Read the model definition and answer for the solid it produces. Units are mm, in the model's axes. A direction names the side the tool comes from. Coordinates: 2 decimals unless noted, no trailing zeros. Order: outer loops, then holes, each group sorted by start corner. A loop starts at its lowest first (then second) coordinate and runs counter-clockwise, first axis right, second up. Notation, with made-up numbers: M 3.25,-23 L 55.25,-23 A20 cw 55.25,-12 Z; hole C 31,-37 d1. An arc over 180 degrees is marked long. Write each question's results on one line, items separated by ' | '.
```python
from build123d import *

# Parameters (mm, degrees)
F0_W           = 29
F0_H           = 35
F0_R           = 1.15
F0_W_2         = 19
F0_H_2         = 25
F1_DEPTH       = 6.5
F2_W           = 29
F2_H           = 35
F2_R           = 1.15
F2_W_2         = 19
F2_H_2         = 25
F3_DEPTH       = 4
F4_W           = 11
F4_H           = 5
F4_W_2         = 5
F5_DEPTH       = 6
F6_R           = 2
F8_D           = 2.9
F8_CBORE_D     = 5.5
F8_CBORE_DEPTH = 2.5


with BuildPart() as f1:
    # F0 (on Top) → F1 (new body)
    with BuildSketch(Plane.XY):
        Rectangle(F0_W, F0_H)
        with Locations((-12, -15)):
            Circle(F0_R, mode=Mode.SUBTRACT)
        with Locations((12, -15)):
            Circle(F0_R, mode=Mode.SUBTRACT)
        with Locations((-12, 15)):
            Circle(F0_R, mode=Mode.SUBTRACT)
        Rectangle(F0_W_2, F0_H_2, mode=Mode.SUBTRACT)
        with Locations((12, 15)):
            Circle(F0_R, mode=Mode.SUBTRACT)
    extrude(amount=F1_DEPTH)

    # F2 (on face) → F3 (join)
    with BuildSketch(Plane(origin=(0, 0, 0), x_dir=(1, 0, 0), z_dir=(0, 0, -1))):
        Rectangle(F2_W, F2_H)
        with Locations((-12, -15)):
            Circle(F2_R, mode=Mode.SUBTRACT)
        with Locations((12, -15)):
            Circle(F2_R, mode=Mode.SUBTRACT)
        with Locations((-12, 15)):
            Circle(F2_R, mode=Mode.SUBTRACT)
        Rectangle(F2_W_2, F2_H_2, mode=Mode.SUBTRACT)
        with Locations((12, 15)):
            Circle(F2_R, mode=Mode.SUBTRACT)
        with Locations((-12, 15)):
            Circle(F2_R)
        with Locations((12, 15)):
            Circle(F2_R)
        with Locations((-12, -15)):
            Circle(F2_R)
        Rectangle(F2_W_2, F2_H_2)
        with Locations((12, -15)):
            Circle(F2_R)
    extrude(amount=F3_DEPTH)

    # F4 (on face) → F5 (cut)
    with BuildSketch(Plane.XY.offset(6.5)):
        with Locations((0, -15)):
            Rectangle(F4_W, F4_H)
        with Locations((0, 15)):
            Rectangle(F4_W_2, F4_H)
    extrude(amount=-F5_DEPTH, mode=Mode.SUBTRACT)

    # F6
    f6_edges = [f1.edges().sort_by_distance(p)[0] for p in [
        (-14.5, 17.5, 1.25),
        (14.5, 17.5, 1.25),
        (14.5, -17.5, 1.25),
        (-14.5, -17.5, 1.25),
    ]]
    fillet(f6_edges, radius=F6_R)

    # F8 (through all)
    with Locations(Plane.XY):
        with Locations((0, 7), (0, -7)):
            CounterBoreHole(F8_D / 2, F8_CBORE_D / 2, F8_CBORE_DEPTH)


solid = f1.part
```
(1) The part is cut by section A-A, the plane z = 2.75. Write down the section's boundary in (x, y), then the cut area to 3 significant figures.
Conclusion:
outline: M -14.5,-15.5 A2 ccw -12.5,-17.5 L -5.5,-17.5 L -5.5,-12.5 L -9.5,-12.5 L -9.5,12.5 L -2.5,12.5 L -2.5,17.5 L -12.5,17.5 A2 ccw -14.5,15.5 Z; M 2.5,12.5 L 9.5,12.5 L 9.5,-12.5 L 5.5,-12.5 L 5.5,-17.5 L 12.5,-17.5 A2 ccw 14.5,-15.5 L 14.5,15.5 A2 ccw 12.5,17.5 L 2.5,17.5 Z; hole C -12,-15 d2.3; hole C -12,15 d2.3; hole C 12,-15 d2.3; hole C 12,15 d2.3 | area: 440 mm²
(2) The part is cut by section B-B, the plane y = -7. Write down the section's boundary in (x, z), then the cut area to 3 significant figures.
Conclusion:
outline: M -14.5,-4 L -1.45,-4 L -1.45,-2.5 L -2.75,-2.5 L -2.75,0 L -9.5,0 L -9.5,6.5 L -14.5,6.5 Z; M 1.45,-4 L 14.5,-4 L 14.5,6.5 L 9.5,6.5 L 9.5,0 L 2.75,0 L 2.75,-2.5 L 1.45,-2.5 Z | area: 163 mm²
(3) Straight lines are drawn through the part: line 1 (Y direction, x = 0, z = -3.4); line 2 (Y direction, x = 0, z = -1.15); line 3 (Y direction, x = 6.75, z = 2.25). For each, find the intervals that lie inside material, in ascending order.
Conclusion:
line 1: -17.5 to -8.45, -5.55 to 5.55, 8.45 to 17.5 | line 2: -17.5 to -9.75, -4.25 to 4.25, 9.75 to 17.5 | line 3: -17.5 to -12.5, 12.5 to 17.5
(4) For faces 1 (the flat face through (0, 15, 0.5)), 2 (the flat face through (1.2, -8.2, -2.5)), 3 (the flat face through (-5.5, -15, 4)), determine the directions among +Z, -Z, +X, -X, +Y, -Y from which every point of the face is accessible in a straight line to the end or side of a thin tool.
Conclusion:
face 1: +Z, +Y, -Y | face 2: +Z | face 3: +Z, -Y
(5) Given pin 1 (4.5 mm diameter, centred on x = 0, y = 7, fed in from +Z); pin 2 (1.1 mm diameter, centred on x = 12.5, y = 15, fed in from +Z); pin 3 (2.5 mm diameter, centred on x = -12, y = -15.5, fed in from +Z); pin 4 (2.5 mm diameter, centred on x = 1, y = 15.5, fed in from +Z), each flat-ended and moving along its own axis, determine where each tip first touches the part or whether it passes through.
Conclusion:
pin 1: z = -2.5 | pin 2: z = 0 | pin 3: z = 6.5 | pin 4: z = 0.5
(6) The part is cut by section D-D, the plane z = -1.5. Write down the section's boundary in (x, y), then the cut area to 3 significant figures.
Conclusion:
outline: M -14.5,-15.5 A2 ccw -12.5,-17.5 L 12.5,-17.5 A2 ccw 14.5,-15.5 L 14.5,15.5 A2 ccw 12.5,17.5 L -12.5,17.5 A2 ccw -14.5,15.5 Z; hole C 0,-7 d5.5; hole C 0,7 d5.5 | area: 964 mm²
(7) The part is cut by section C-C, the plane x = 0. Write down the section's boundary in (y, z).
Conclusion:
outline: M -17.5,-4 L -8.45,-4 L -8.45,-2.5 L -9.75,-2.5 L -9.75,0 L -12.5,0 L -12.5,0.5 L -17.5,0.5 Z; M -5.55,-4 L 5.55,-4 L 5.55,-2.5 L 4.25,-2.5 L 4.25,0 L -4.25,0 L -4.25,-2.5 L -5.55,-2.5 Z; M 8.45,-4 L 17.5,-4 L 17.5,0.5 L 12.5,0.5 L 12.5,0 L 9.75,0 L 9.75,-2.5 L 8.45,-2.5 Z
